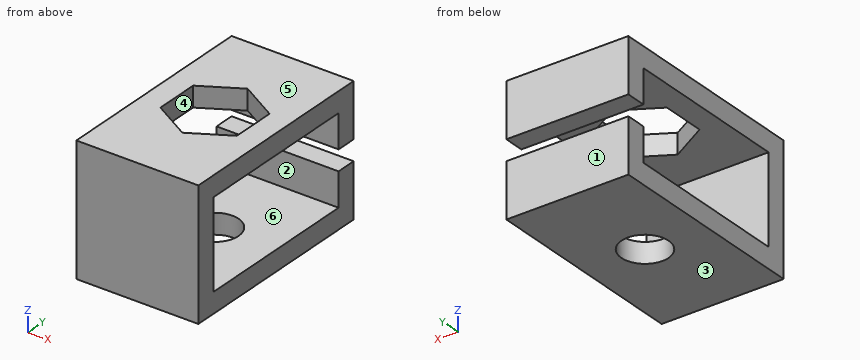
```python
from build123d import *

# Parameters (mm, degrees)
TOP_START                      = -3.123265701
TOP_BAR_CUT_EXTRUDE1_OUTLINE_W = 203.2
TOP_BAR_CUT_EXTRUDE1_OUTLINE_H = 25.4
TOP_BAR_CUT_EXTRUDE1_DEPTH     = 12.7
TOP_START_2                    = 6.35
TOP_BAR_OUTLINE_W              = 203.2
TOP_BAR_OUTLINE_H              = 25.4
TOP_BAR_DEPTH                  = 3.226734299
TOP_BAR_2_DEPTH                = 9.473265701
TOP_START_3                    = -6.35
TOP_BAR_3_OUTLINE_W            = 203.2
TOP_BAR_3_OUTLINE_H            = 25.4
TOP_BAR_3_DEPTH                = 12.7
BOSS_EXTRUDE2_DEPTH            = 9.525
SKETCH4_R                      = 3.675
CUT_EXTRUDE1_DEPTH             = 28.583849441
CUT_EXTRUDE2_DEPTH             = 3.175


# Read off the part's stored shape, not the designer's step: <top bar>-<Cut-Extrude1>, top bar
with BuildPart() as part:
    # <top bar>-<Cut-Extrude1> outline → <top bar>-<Cut-Extrude1> (new body)
    with BuildSketch(Plane.XY.offset(TOP_START)):
        with Locations((-0.022421442, 2.056236138)):
            Rectangle(TOP_BAR_CUT_EXTRUDE1_OUTLINE_W, TOP_BAR_CUT_EXTRUDE1_OUTLINE_H)
        with BuildLine():
            ThreePointArc((-95.272421442, -1.618763862), (-98.947421442, 2.056236138), (-95.272421442, 5.731236138))
            Line((-95.272421442, 5.731236138), (6.327578558, 5.731236138))
            ThreePointArc((6.327578558, 5.731236138), (10.002578558, 2.056236138), (6.327578558, -1.618763862))
            Line((6.327578558, -1.618763862), (-95.272421442, -1.618763862))
        make_face(mode=Mode.SUBTRACT)
    extrude(amount=TOP_BAR_CUT_EXTRUDE1_DEPTH)

    # top bar outline → top bar (cut)
    with BuildSketch(Plane.XY.offset(TOP_START_2)):
        with Locations((-0.022421442, 2.056236138)):
            Rectangle(TOP_BAR_OUTLINE_W, TOP_BAR_OUTLINE_H)
        with BuildLine():
            ThreePointArc((6.327578558, 5.731236138), (10.002578558, 2.056236138), (6.327578558, -1.618763862))
            Line((6.327578558, -1.618763862), (-95.272421442, -1.618763862))
            ThreePointArc((-95.272421442, -1.618763862), (-98.947421442, 2.056236138), (-95.272421442, 5.731236138))
            Line((-95.272421442, 5.731236138), (6.327578558, 5.731236138))
        make_face(mode=Mode.SUBTRACT)
    extrude(amount=TOP_BAR_DEPTH, mode=Mode.SUBTRACT)

    # top bar 2 outline → top bar 2 (cut)
    with BuildSketch(Plane.XY.offset(TOP_START)):
        Polygon((-101.6, 12.7), (101.577578558, 12.7), (101.577578558, 14.756236138), (-101.622421442, 14.756236138), (-101.622421442, -10.643763862), (-101.6, -10.643763862), align=None)
        with BuildLine():
            ThreePointArc((-95.272421442, -1.618763862), (-97.461703705, -0.895486778), (-98.789240286, 0.989648017))
            ThreePointArc((-98.789240286, 0.989648017), (-98.177676678, -2.221336145), (-95.25, -3.675))
            Line((-95.25, -3.675), (6.35, -3.675))
            ThreePointArc((6.35, -3.675), (9.301722916, -2.189282263), (9.866818844, 1.066588121))
            ThreePointArc((9.866818844, 1.066588121), (8.548914703, -0.87144054), (6.327578558, -1.618763862))
            Line((6.327578558, -1.618763862), (-95.272421442, -1.618763862))
        make_face()
    extrude(amount=TOP_BAR_2_DEPTH, mode=Mode.SUBTRACT)

    # top bar 3 outline → top bar 3 (add)
    with BuildSketch(Plane.XY.offset(TOP_START_3)):
        Rectangle(TOP_BAR_3_OUTLINE_W, TOP_BAR_3_OUTLINE_H)
        with BuildLine():
            ThreePointArc((-95.25, -3.675), (-98.925, 0), (-95.25, 3.675))
            Line((-95.25, 3.675), (6.35, 3.675))
            ThreePointArc((6.35, 3.675), (10.025, 0), (6.35, -3.675))
            Line((6.35, -3.675), (-95.25, -3.675))
        make_face(mode=Mode.SUBTRACT)
    extrude(amount=TOP_BAR_3_DEPTH)


with BuildPart() as body_2:
    # Sketch3 → Boss-Extrude2 (new, symmetric)
    with BuildSketch(Plane(origin=(0, 0, 0), x_dir=(0, 0, -1), z_dir=(1, 0, 0))):
        Polygon((-1.5875, 13.2), (-1.5875, 16.375), (-10.025, 16.375), (-10.025, -16.375), (10.025, -16.375), (10.025, 16.375), (1.5875, 16.375), (1.5875, 13.2), (6.85, 13.2), (6.85, -13.2), (-6.85, -13.2), (-6.85, 13.2), align=None)
    extrude(amount=BOSS_EXTRUDE2_DEPTH, both=True)

    # Sketch4 → Cut-Extrude1 (cut, through all)
    with BuildSketch(Plane(origin=(0, 0, -10.025), x_dir=(-1, 0, 0), z_dir=(0, 0, -1))):
        with Locations(Location((0, 0, 0), (0, 0, 90))):
            Circle(SKETCH4_R)
    extrude(amount=-CUT_EXTRUDE1_DEPTH, mode=Mode.SUBTRACT)

    # Sketch5 → Cut-Extrude2 (cut)
    with BuildSketch(Plane.XY.offset(10.025)):
        Polygon((0, 6.892407514), (-5.969, 3.446203757), (-5.969, -3.446203757), (0, -6.892407514), (5.969, -3.446203757), (5.969, 3.446203757), align=None)
    extrude(amount=-CUT_EXTRUDE2_DEPTH, mode=Mode.SUBTRACT)


solid = body_2.part
```
The model under review builds one solid part; all positions refer to its coordinate system, in mm. Face numbers are marked on the shaded views. A direction names the side the tool comes from. Round coordinates to 2 decimals unless told otherwise and drop trailing zeros. Order: outer loops, then holes, each group sorted by start corner. A loop starts at its lowest first (then second) coordinate and runs counter-clockwise, first axis right, second up.
(1) Take a section at A-A, the plane y = 11. State the section outline as (x, z) points (3 decimals).
Working result:
outline: (-9.525, -10.025) - (9.525, -10.025) - (9.525, -6.85) - (-9.525, -6.85) - close; (-9.525, 6.85) - (9.525, 6.85) - (9.525, 10.025) - (-9.525, 10.025) - close
(2) Wall thickness on L1, parallel to Z at x = 6.5, y = -12 (3 decimals); L2, parallel to Y at x = -0.5, z = -2.25 (3 decimals); L3, parallel to Z at x = 5.75, y = 14.5 (1 decimal): over which ranges is each line inside the solid? List them lowest first.
Working result:
L1: z = -10.025 to -6.85, 6.85 to 10.025
L2: y = -16.375 to -13.2, 13.2 to 16.375
L3: z = -10 to -1.6, 1.6 to 10
(3) Tool access review of the marked faces 4, 5 and 6: name each direction out of +Z, -Z, +X, -X, +Y, -Y from which nothing blocks a thin tool from reaching the whole face with its end or side.
Working result:
face 4: +Z
face 5: +Z, +X, -X, +Y, -Y
face 6: +X, -X
(4) For P1, Ø12, axis at y = -9, z = 2, coming from the -X side (3 decimals); P2, Ø5.5, axis at x = 0.5, y = -2.5, coming from the +Z side, all flat-tipped, find the tip position at first contact; note any pin that passes through.
Working result:
P1: stops at x = -9.525
P2: stops at z = -6.85
(5) Mouldability with a two-part tool opening along Z and no side actions: class the marked faces 1, 2 and 3 as released by +Z, released by -Z, zero draft, split by the parting line, or undercut.
Working result:
face 1: zero draft
face 2: undercut
face 3: released by -Z
(6) Take a section at B-B, the plane z = 5.25. State the section outline as (x, y) points (3 decimals), plus the area to 3 significant figures.
Working result:
outline: (-9.525, -16.375) - (9.525, -16.375) - (9.525, -13.2) - (-9.525, -13.2) - close; (-9.525, 13.2) - (9.525, 13.2) - (9.525, 16.375) - (-9.525, 16.375) - close
area: 121 mm2
(7) Take a section at C-C, the plane y = 0. State the section outline as (x, z) points (3 decimals).
Working result:
outline: (-9.525, -10.025) - (-3.675, -10.025) - (-3.675, -6.85) - (-9.525, -6.85) - close; (-9.525, 6.85) - (-5.969, 6.85) - (-5.969, 10.025) - (-9.525, 10.025) - close; (3.675, -10.025) - (9.525, -10.025) - (9.525, -6.85) - (3.675, -6.85) - close; (5.969, 6.85) - (9.525, 6.85) - (9.525, 10.025) - (5.969, 10.025) - close
